from build123d import *

# Parameters (mm, degrees)
CROQUIS1_R                 = 3
SALIENTE_EXTRUIR1_DEPTH    = 51
CORTAR_EXTRUIR1_DEPTH      = 311.888957589
CORTAR_EXTRUIR1_DEPTH_BACK = 311.888957589
CROQUIS2_W                 = 181.964548074
CROQUIS2_H                 = 27.905532643
CROQUIS2_W_2               = 174.878216902
CROQUIS2_H_2               = 60.347618799
CROQUIS2_W_3               = 330
CROQUIS2_H_3               = 10


with BuildPart() as part:
    # Croquis1 → Saliente-Extruir1 (new body)
    # profile 1 of 4: a face of its own
    with BuildSketch(Plane.XY):
        with BuildLine():
            Line((141.907724078, 74.393898239), (106.962723162, 58.37688333))
            ThreePointArc((106.962723162, 58.37688333), (116.54115135, 54.372948072), (115.362717192, 44.058439988))
            ThreePointArc((115.362717192, 44.058439988), (114.912044927, 43.584270047), (114.45954291, 43.111845929))
            Line((114.45954291, 43.111845929), (141.660745717, 55.579496794))
            ThreePointArc((141.660745717, 55.579496794), (163.715018222, 45.838294791), (185.769290727, 55.579496794))
            ThreePointArc((185.769290727, 55.579496794), (210.289811625, 39.891989826), (236.56917478, 52.411929606))
            ThreePointArc((236.56917478, 52.411929606), (262.563049751, 34.849044969), (290.598242925, 48.926132611))
            ThreePointArc((290.598242925, 48.926132611), (291.527530464, 63.45988081), (281.907724078, 74.393898239))
            add(Edge.make_bspline(
                [(141.907724078, 74.393898239), (211.705167047, 100.839206128), (281.907724078, 74.393898239)],
                knots=[0, 0, 0, 1, 1, 1], degree=2))
        make_face()
    # profile 2 of 4: a face of its own
    with BuildSketch(Plane.XY):
        with BuildLine():
            ThreePointArc((105.545350362, 57.727231572), (116.814352718, 53.541770784), (112.62889193, 42.272768428))
            Line((112.62889193, 42.272768428), (114.45954291, 43.111845929))
            ThreePointArc((114.45954291, 43.111845929), (114.912044927, 43.584270047), (115.362717192, 44.058439988))
            ThreePointArc((115.362717192, 44.058439988), (116.54115135, 54.372948072), (106.962723162, 58.37688333))
            Line((106.962723162, 58.37688333), (105.545350362, 57.727231572))
        make_face()
    # profile 3 of 4: a face of its own
    with BuildSketch(Plane.XY):
        with BuildLine():
            Line((-2.124397984, 8.37688333), (-3.541770784, 7.727231572))
            ThreePointArc((-3.541770784, 7.727231572), (-7.727231572, -3.541770784), (3.541770784, -7.727231572))
            Line((3.541770784, -7.727231572), (112.62889193, 42.272768428))
            ThreePointArc((112.62889193, 42.272768428), (116.814352718, 53.541770784), (105.545350362, 57.727231572))
            Line((105.545350362, 57.727231572), (104.127977562, 57.077579814))
            ThreePointArc((104.127977562, 57.077579814), (103.441106721, 56.542764112), (102.8115251, 55.941560012))
            ThreePointArc((102.8115251, 55.941560012), (55.789043947, 22.282676087), (-0.404455893, 8.63259269))
            ThreePointArc((-0.404455893, 8.63259269), (-1.270874621, 8.548106154), (-2.124397984, 8.37688333))
        make_face()
        Circle(CROQUIS1_R, mode=Mode.SUBTRACT)
        with Locations((109.087121146, 50)):
            Circle(CROQUIS1_R, mode=Mode.SUBTRACT)
    # profile 4 of 4: a face of its own
    with BuildSketch(Plane.XY):
        with BuildLine():
            ThreePointArc((3.541770784, -7.727231572), (-7.727231572, -3.541770784), (-3.541770784, 7.727231572))
            Line((-3.541770784, 7.727231572), (-2.124397984, 8.37688333))
            ThreePointArc((-2.124397984, 8.37688333), (-8.548106154, -1.270874621), (0.404455893, -8.63259269))
            ThreePointArc((0.404455893, -8.63259269), (62.395554487, 6.298958939), (114.45954291, 43.111845929))
            Line((114.45954291, 43.111845929), (112.62889193, 42.272768428))
            Line((112.62889193, 42.272768428), (3.541770784, -7.727231572))
        make_face()
    extrude(amount=SALIENTE_EXTRUIR1_DEPTH)

    # Croquis2 → Cortar-Extruir1 (cut, two sides: drawn at the far end of the back side and taken through both)
    with BuildSketch(Plane(origin=(-3.541770784, 7.727231572, 0), x_dir=(0.9090593428863096, 0.4166666666666667, 0), z_dir=(-0.41666666666666663, 0.9090593428863095, 0)).offset(-CORTAR_EXTRUIR1_DEPTH_BACK)):
        with Locations((65.517476081, 3.452766322)):
            Rectangle(CROQUIS2_W, CROQUIS2_H)
        with Locations((69.060641667, -70.6738094)):
            Rectangle(CROQUIS2_W_2, CROQUIS2_H_2)
        with Locations((-8.500249882, -25.5)):
            Rectangle(CROQUIS2_W_3, CROQUIS2_H_3)
    extrude(amount=CORTAR_EXTRUIR1_DEPTH + CORTAR_EXTRUIR1_DEPTH_BACK, mode=Mode.SUBTRACT)


solid = part.part
Work out the finished part from the listing and answer in its coordinate system (mm). A direction names the side the tool comes from. Round coordinates to 2 decimals unless told otherwise and drop trailing zeros. Order: outer loops, then holes, each group sorted by start corner. A loop starts at its lowest first (then second) coordinate and runs counter-clockwise, first axis right, second up. Notation, with made-up numbers: M 21.25,61.5 L 58.25,61.5 A17 cw 58.25,86.5 Z; hole C -22,79 d4. An arc over 180 degrees is marked long. Put each result on its own line as item: value. Start each with the question number.
Q1. A tool of negligible diameter and unlimited length cuts with its end or side. For faces 4 (the flat face through (144.184, 61.027, 25.57)), 5 (the flat face through (215, 61, 51)), 6 (the flat face through (144.184, 61.027, 5.323)), 7 (the cylindrical face through (-3, 0, 15)), 8 (the flat face through (127.87, 49.26, 15.43)), from which of +Z, -Z, +X, -X, +Y, -Y can it reach the whole face along a straight path? Write none if from no direction.
Q2. Section A-A, the plane y = 0 is taken. Write down the section's boundary in (x, z).
Q3. Flat-ended cylindrical pins translate along their axes: pin 1 (5 mm diameter, centred on x = 118, y = 49, fed in from +Z); pin 2 (3.5 mm diameter, centred on x = 109.09, y = 50, fed in from +Z); pin 3 (1.5 mm diameter, centred on x = 227, z = 45.5, fed in from -Y); pin 4 (12 mm diameter, centred on x = 42, z = 9, fed in from -Y). Find the tip coordinate at first contact, or state that the pin passes through.
Q4. Straight lines are drawn through the part: L1, parallel to Y at x = 0, z = 36.75; L2, parallel to X at y = 50, z = 16; L3, parallel to Z at x = 135, y = 62. For each, find the intervals that lie inside material, in ascending order. Write a range as [from, to].
Q5. Section C-C, the plane z = 14.5 is taken. Give the number of separate pieces and of enclosed holes in the cut face, and give its area (3 significant figures).
Q6. For a pull along X with two mould halves and no side action, classify faces 1 (the cylindrical face through (106.88, 52.03, 35.43)), 2 (the flat face through (215, 61, 0)), 3 (the cylindrical face through (56.529, 22.624, 35.43)) as pulls with the +X half, pulls with the -X half, needs draft (parallel to the pull), parting line crosses it, or undercut.
Q7. Section B-B, the plane y = 31.5 is taken. Write down the section's boundary in (x, z), and give its area (3 significant figures).
Findings below:
1. face 4: -X, -Y
1. face 5: +Z, +X, -X, +Y, -Y
1. face 6: -Z, -X, -Y
1. face 7: +Z, -Z
1. face 8: +Z, -Z, -Y
2. outline: M -8.64,10.5 L -3,10.5 L -3,20.5 L -8.64,20.5 Z; M -8.64,30.5 L -3,30.5 L -3,40.5 L -8.64,40.5 Z; M 3,10.5 L 46.4,10.5 L 46.4,20.5 L 3,20.5 Z; M 3,30.5 L 46.4,30.5 L 46.4,40.5 L 3,40.5 Z
3. pin 1: stops at z = 40.5
3. pin 2: passes through
3. pin 3: stops at y = 43.35
3. pin 4: stops at y = -3.08
4. L1: y = [-8.64, -3], [3, 8.65]
4. L2: x = [96.87, 106.09], [112.09, 129.49], [148.52, 178.91], [189.66, 234.66], [237.86, 291.08]
4. L3: z = [10.5, 20.5], [30.5, 40.5]
5. separate pieces: 1
5. enclosed holes: 2
5. area: 8,590 mm^2
6. face 1: undercut
6. face 2: needs draft
6. face 3: pulls with the -X half
7. outline: M 72.91,10.5 L 102.12,10.5 L 102.12,20.5 L 72.91,20.5 Z; M 72.91,30.5 L 102.12,30.5 L 102.12,40.5 L 72.91,40.5 Z
7. area: 584 mm^2
